Read the model definition and answer for the solid it produces. Units are mm, in the model's axes. A direction names the side the tool comes from. Give positions to 0.01 mm unless a question says otherwise; leave off trailing zeros. Order: outer loops, then holes, each group sorted by start corner. A loop starts at its lowest first (then second) coordinate and runs counter-clockwise, first axis right, second up. Notation, with made-up numbers: (17, -31) -> (75, -31) arc R17 ccw to (75, 2) -> close; hole circle Ø8 at (-2, -6). An arc over 180 degrees is marked (long way). Use one line per item in the form item = value.
```python
from build123d import *

# Parameters (mm, degrees)
SKETCH1_W           = 26
SKETCH1_H           = 24
BOSS_EXTRUDE1_DEPTH = 0.7
SKETCH2_W           = 2
SKETCH2_H           = 22
BOSS_EXTRUDE2_DEPTH = 1.3
CUT_EXTRUDE2_DEPTH  = 0.4
SKETCH4_W           = 1
SKETCH4_H           = 24
BOSS_EXTRUDE3_DEPTH = 0.7


with BuildPart() as part:
    # Sketch1 → Boss-Extrude1 (new body)
    with BuildSketch(Plane(origin=(0, 0, 0), x_dir=(1, 0, 0), z_dir=(0, 1, 0))):
        Rectangle(SKETCH1_W, SKETCH1_H)
    extrude(amount=BOSS_EXTRUDE1_DEPTH)

    # Sketch2 → Boss-Extrude2 (add)
    with BuildSketch(Plane(origin=(0, 0.7, 0), x_dir=(1, 0, 0), z_dir=(0, 1, 0))):
        with Locations((11, 0)):
            Rectangle(SKETCH2_W, SKETCH2_H)
    extrude(amount=BOSS_EXTRUDE2_DEPTH)

    # Sketch3 → Cut-Extrude2 (cut)
    with BuildSketch(Plane(origin=(0, 0.7, 0), x_dir=(1, 0, 0), z_dir=(0, 1, 0))):
        with BuildLine():
            Line((-2.366025404, 7.5), (-11.026279442, -7.5))
            ThreePointArc((-11.026279442, -7.5), (-11.026279442, -8.5), (-10.160254038, -9))
            Line((-10.160254038, -9), (7.160254038, -9))
            ThreePointArc((7.160254038, -9), (8.026279442, -8.5), (8.026279442, -7.5))
            Line((8.026279442, -7.5), (-0.633974596, 7.5))
            ThreePointArc((-0.633974596, 7.5), (-1.5, 8), (-2.366025404, 7.5))
        make_face()
    extrude(amount=-CUT_EXTRUDE2_DEPTH, mode=Mode.SUBTRACT)

    # Sketch4 → Boss-Extrude3 (add)
    with BuildSketch(Plane(origin=(0, 0.7, 0), x_dir=(1, 0, 0), z_dir=(0, 1, 0))):
        with Locations((-13.5, 0)):
            Rectangle(SKETCH4_W, SKETCH4_H)
    extrude(amount=-BOSS_EXTRUDE3_DEPTH)


solid = part.part
```
Item 1: The part is cut by section B-B on x = -6.75. Give the vertices of the cut face in (y, z), and give its area (3 significant figures).
Checks:
outline = (0, -12) -> (0.7, -12) -> (0.7, 0.09) -> (0.3, 0.09) -> (0.3, 9) -> (0.7, 9) -> (0.7, 12) -> (0, 12) -> close
area = 13.2 mm²
Item 2: The part is cut by section D-D on z = -3.5. Give the vertices of the cut face in (x, y), and give its area (3 significant figures).
Checks:
outline = (-14, 0) -> (13, 0) -> (13, 0.7) -> (12, 0.7) -> (12, 2) -> (10, 2) -> (10, 0.7) -> (1.68, 0.7) -> (1.68, 0.3) -> (-4.68, 0.3) -> (-4.68, 0.7) -> (-14, 0.7) -> close
area = 19.0 mm²
Item 3: Which of the six approach directions +Z, -Z, +X, -X, +Y, -Y give full straight-line access (tool end or side, diameter ignored) to faces 1 (the flat face through (11, 2, 0)), 2 (the flat face through (3.757, 0.503, 0.105)), 3 (the flat face through (11, 1, -11)), 4 (the flat face through (12, 1, 0)), 5 (the flat face through (10, 1, 0))?
Checks:
face_1 = +Z, -Z, +X, -X, +Y
face_2 = +Y
face_3 = -Z, +X, -X, +Y
face_4 = +Z, -Z, +X, +Y
face_5 = +Z, -Z, -X, +Y
Item 4: The part is cut by section A-A on z = -9. Give the vertices of the cut face in (x, y).
Checks:
outline = (-14, 0) -> (13, 0) -> (13, 0.7) -> (12, 0.7) -> (12, 2) -> (10, 2) -> (10, 0.7) -> (-14, 0.7) -> close
Item 5: Given pin 1 Ø3 at (x, z) = (4, -5.5) entering from +Y; pin 2 Ø1 at (x, y) = (11.5, 1.5) entering from +Z; pin 3 Ø5 at (x, z) = (-2.5, 1.5) entering from +Y, each flat-ended and moving along its own axis, determine where each tip first touches the part or whether it passes through.
Checks:
pin_1 = 0.7
pin_2 = 11
pin_3 = 0.3
Item 6: Straight lines are drawn through the part: L1, parallel to X at y = 1.1, z = 5.75; L2, parallel to Y at x = 3.75, z = 10.25; L3, parallel to Z at x = 11.25, y = 1.7. For each, find the intervals that lie inside material, in ascending order. Write a range as from..to.
Checks:
L1 = 10..12
L2 = 0..0.7
L3 = -11..11
Item 7: The part is cut by section C-C on y = 1.6. Give the vertices of the cut face in (x, z), and give its area (3 significant figures).
Checks:
outline = (10, -11) -> (12, -11) -> (12, 11) -> (10, 11) -> close
area = 44.0 mm²
Item 8: Determine the mould class of faces 6 (the flat face through (-1, 0, 0)), 7 (the cylindrical face through (-11.03, 0.5, 8.49)), 8 (the flat face through (11, 1, 11)) for opening direction Z: +Z half, -Z half, draft (parallel to the pull), parting line (faces both ways), or undercut.
Checks:
face_6 = draft
face_7 = undercut
face_8 = +Z half
